```python
from build123d import *

# Parameters (mm, degrees)
SKETCH_W        = 100.5
SKETCH_H        = 50
SKETCH_R        = 19
SKETCH_R_2      = 1.7
SKETCH_W_2      = 20
SKETCH_H_2      = 40
PAD_DEPTH       = 8
SKETCH001_W     = 86.5
SKETCH001_H     = 44
POCKET_DEPTH    = 3
SKETCH002_W     = 96.5
SKETCH002_H     = 2
POCKET001_DEPTH = 4
POCKET002_DEPTH = 2.5
PAD001_DEPTH    = 53
SKETCH005_R     = 1.5
POCKET003_DEPTH = 30
SKETCH006_R     = 1.7
POCKET004_DEPTH = 50.001
POCKET006_DEPTH = 2
FILLET_R        = 3
FILLET001_R     = 3
FILLET002_R     = 3
FILLET003_R     = 3
CHAMFER_SIZE    = 1.6
CHAMFER001_SIZE = 1.6
CHAMFER002_SIZE = 1.6
CHAMFER003_SIZE = 1.6


with BuildPart() as part:
    # Sketch → Pad (new body)
    with BuildSketch(Plane.XY):
        Rectangle(SKETCH_W, SKETCH_H)
        with Locations((23.25, 0)):
            Circle(SKETCH_R, mode=Mode.SUBTRACT)
        with Locations((7.25, 16)):
            Circle(SKETCH_R_2, mode=Mode.SUBTRACT)
        with Locations((39.25, 16)):
            Circle(SKETCH_R_2, mode=Mode.SUBTRACT)
        with Locations((39.25, -16)):
            Circle(SKETCH_R_2, mode=Mode.SUBTRACT)
        with Locations((7.25, -16)):
            Circle(SKETCH_R_2, mode=Mode.SUBTRACT)
        with Locations((-8, 16)):
            Circle(SKETCH_R_2, mode=Mode.SUBTRACT)
        with Locations((-8, -16)):
            Circle(SKETCH_R_2, mode=Mode.SUBTRACT)
        with Locations((-24.25, 0)):
            Rectangle(SKETCH_W_2, SKETCH_H_2, mode=Mode.SUBTRACT)
    extrude(amount=PAD_DEPTH)

    # Sketch001 → Pocket (cut)
    with BuildSketch(Plane.XY.offset(8)):
        Rectangle(SKETCH001_W, SKETCH001_H)
    extrude(amount=-POCKET_DEPTH, mode=Mode.SUBTRACT)

    # Sketch002 → Pocket001 (cut)
    with BuildSketch(Plane.XY.offset(8)):
        with Locations((0, 10.5)):
            Rectangle(SKETCH002_W, SKETCH002_H)
        with Locations((0, -4.5)):
            Rectangle(SKETCH002_W, SKETCH002_H)
    extrude(amount=-POCKET001_DEPTH, mode=Mode.SUBTRACT)

    # Sketch003 → Pocket002 (cut)
    with BuildSketch(Plane.XY.offset(5)):
        Polygon((6.428139, 19.067226), (4.182774, 16.821861), (5.004634, 13.754634), (8.071861, 12.932774), (10.317226, 15.178139), (9.495366, 18.245366), align=None)
        Polygon((40.071861, 19.067226), (37.004634, 18.245366), (36.182774, 15.178139), (38.428139, 12.932774), (41.495366, 13.754634), (42.317226, 16.821861), align=None)
        Polygon((5.004634, -13.754634), (4.182774, -16.821861), (6.428139, -19.067226), (9.495366, -18.245366), (10.317226, -15.178139), (8.071861, -12.932774), align=None)
        Polygon((36.182774, -15.178139), (37.004634, -18.245366), (40.071861, -19.067226), (42.317226, -16.821861), (41.495366, -13.754634), (38.428139, -12.932774), align=None)
        Polygon((-9.587713, 18.75), (-11.175426, 16), (-9.587713, 13.25), (-6.412287, 13.25), (-4.824574, 16), (-6.412287, 18.75), align=None)
        Polygon((-9.587713, -13.25), (-11.175426, -16), (-9.587713, -18.75), (-6.412287, -18.75), (-4.824574, -16), (-6.412287, -13.25), align=None)
    extrude(amount=-POCKET002_DEPTH, mode=Mode.SUBTRACT)

    # Sketch004 → Pad001 (new body)
    with BuildSketch(Plane.XY.offset(8)):
        Polygon((-50.25, 25), (50.25, 25), (50.25, 17), (43.25, 17), (43.25, 22), (-43.25, 22), (-43.25, 17), (-50.25, 17), align=None)
        Polygon((50.25, -17), (50.25, -25), (-50.25, -25), (-50.25, -17), (-43.25, -17), (-43.25, -22), (43.25, -22), (43.25, -17), align=None)
    extrude(amount=PAD001_DEPTH)

    # Sketch005 → Pocket003 (cut)
    with BuildSketch(Plane.XY.offset(61)):
        with Locations((-47, 21)):
            Circle(SKETCH005_R)
        with Locations((47, 21)):
            Circle(SKETCH005_R)
        with Locations((47, -21)):
            Circle(SKETCH005_R)
        with Locations((-47, -21)):
            Circle(SKETCH005_R)
    extrude(amount=-POCKET003_DEPTH, mode=Mode.SUBTRACT)

    # Sketch006 → Pocket004 (cut, through all)
    with BuildSketch(Plane(origin=(0, 25, 0), x_dir=(-1, 0, 0), z_dir=(0, 1, 0))):
        with Locations((-18, 20)):
            Circle(SKETCH006_R)
        with Locations((18, 20)):
            Circle(SKETCH006_R)
        with Locations((-18, 40)):
            Circle(SKETCH006_R)
        with Locations((18, 40)):
            Circle(SKETCH006_R)
    extrude(amount=-POCKET004_DEPTH, mode=Mode.SUBTRACT)

    # Sketch008 → Pocket006 (cut)
    with BuildSketch(Plane(origin=(0, -22, 0), x_dir=(-1, 0, 0), z_dir=(0, 1, 0))):
        Polygon((-14.824574, 20), (-16.412287, 22.75), (-19.587713, 22.75), (-21.175426, 20), (-19.587713, 17.25), (-16.412287, 17.25), align=None)
        Polygon((21.175426, 20), (19.587713, 22.75), (16.412287, 22.75), (14.824574, 20), (16.412287, 17.25), (19.587713, 17.25), align=None)
        Polygon((-16.412287, 37.25), (-14.824574, 40), (-16.412287, 42.75), (-19.587713, 42.75), (-21.175426, 40), (-19.587713, 37.25), align=None)
        Polygon((19.587713, 37.25), (21.175426, 40), (19.587713, 42.75), (16.412287, 42.75), (14.824574, 40), (16.412287, 37.25), align=None)
    extrude(amount=-POCKET006_DEPTH, mode=Mode.SUBTRACT)

    # Fillet
    fillet_edges = [part.edges().sort_by_distance(p)[0] for p in [
        (-50.25, 25, 34.5),
    ]]
    fillet(fillet_edges, radius=FILLET_R)

    # Fillet001
    fillet001_edges = [part.edges().sort_by_distance(p)[0] for p in [
        (-50.25, -25, 34.5),
    ]]
    fillet(fillet001_edges, radius=FILLET001_R)

    # Fillet002
    fillet002_edges = [part.edges().sort_by_distance(p)[0] for p in [
        (50.25, 25, 34.5),
    ]]
    fillet(fillet002_edges, radius=FILLET002_R)

    # Fillet003
    fillet003_edges = [part.edges().sort_by_distance(p)[0] for p in [
        (50.25, -25, 34.5),
    ]]
    fillet(fillet003_edges, radius=FILLET003_R)

    # Chamfer
    chamfer_edges = [part.edges().sort_by_distance(p)[0] for p in [
        (19.7, 22, 40),
    ]]
    chamfer(chamfer_edges, length=CHAMFER_SIZE)

    # Chamfer001
    chamfer001_edges = [part.edges().sort_by_distance(p)[0] for p in [
        (-16.3, 22, 40),
    ]]
    chamfer(chamfer001_edges, length=CHAMFER001_SIZE)

    # Chamfer002
    chamfer002_edges = [part.edges().sort_by_distance(p)[0] for p in [
        (-16.3, 22, 20),
    ]]
    chamfer(chamfer002_edges, length=CHAMFER002_SIZE)

    # Chamfer003
    chamfer003_edges = [part.edges().sort_by_distance(p)[0] for p in [
        (19.7, 22, 20),
    ]]
    chamfer(chamfer003_edges, length=CHAMFER003_SIZE)


solid = part.part
```
Source: CAD feature listing. Evaluate the final solid. Frame: model axes, mm. A direction names the side the tool comes from. Round coordinates to 2 decimals unless told otherwise and drop trailing zeros. Write each loop counter-clockwise with the first axis right and the second up, starting at its lowest first coordinate (ties: lowest second). Pieces come first, ordered by that corner, then holes. Notation, with made-up numbers: M -8,-0.75 L 23,-0.75 A32 cw 23,34.25 Z; hole C 50,55 d11. An arc over 180 degrees is marked long. Use CSV: the item, a comma, the result in double quotes. Start each with the question number.
Q1. Line query: line 1 (X direction, y = 5.5, z = 3.5); line 2 (Y direction, x = -8, z = 1.85); line 3 (Y direction, x = 7.25, z = 1.4). Output: solid intervals per line, ascending. Write a range as from..to.
Q2. Cut plane B-B on x = -32. Output: boundary loops of the cut face in (y, z).
Q3. Cut plane C-C on z = 13.5. Output: boundary loops of the cut face in (x, y).
Q4. Access query for faces 1 (the face through (18, -23, 17.25)), 2 (the face through (-43.25, 19, 33)), 3 (the face through (47, -17, 34)), 4 (the face through (17.2, -24.5, 38.5)). Directions: +Z, -Z, +X, -X, +Y, -Y. A direction counts if a zero-diameter tool reaches every point of the face in a straight line with its end or side. Return the directions, or none.
Q5. Cut plane D-D on x = -8. Count the separate pieces of the cut face and the enclosed holes in it, plus the area to 4 significant figures.
Q6. First-contact query: P1, Ø3.5, axis at x = -46, y = -5, coming from the +Z side; P2, Ø4.5, axis at x = -7.5, y = -16, coming from the +Z side. Flat tips, straight axial feed; report the tip coordinate or a pass-through.
Q7. Pull-direction query (Y, two-part tool) for faces 5 (the face through (-18.8, 24.3, 38.5)), 6 (the face through (-41, -4, 4)); classes: +Y half, -Y half, draft (parallel to the pull), parting line (faces both ways), or undercut.
Q8. Cut plane A-A on z = 33. Output: boundary loops of the cut face in (x, y), plus the area to 3 significant figures.
Results found:
1,line 1,"-50.25..-34.25, -14.25..5.06, 41.44..50.25"
1,line 2,"-25..-17.7, -14.3..14.3, 17.7..25"
1,line 3,"-25..-17.7, -14.3..-10.25, 10.25..14.3, 17.7..25"
2,outline,"M -25,0 L -20,0 L -20,5 L -22,5 L -22,61 L -25,61 Z; M 20,0 L 25,0 L 25,61 L 22,61 L 22,5 L 20,5 Z"
3,outline,"M -50.25,-22 A3 ccw -47.25,-25 L 47.25,-25 A3 ccw 50.25,-22 L 50.25,-17 L 43.25,-17 L 43.25,-22 L -43.25,-22 L -43.25,-17 L -50.25,-17 Z; M -50.25,17 L -43.25,17 L -43.25,22 L 43.25,22 L 43.25,17 L 50.25,17 L 50.25,22 A3 ccw 47.25,25 L -47.25,25 A3 ccw -50.25,22 Z"
4,face 1,"none"
4,face 2,"+Z"
4,face 3,"+Z, +X, -X"
4,face 4,"+Y, -Y"
5,separate pieces,"3"
5,enclosed holes,"0"
5,area,"537.5 mm^2"
6,P1,"z = 8"
6,P2,"z = 2.5"
7,face 5,"draft"
7,face 6,"undercut"
8,outline,"M -50.25,-22 A3 ccw -47.25,-25 L 47.25,-25 A3 ccw 50.25,-22 L 50.25,-17 L 43.25,-17 L 43.25,-22 L -43.25,-22 L -43.25,-17 L -50.25,-17 Z; M -50.25,17 L -43.25,17 L -43.25,22 L 43.25,22 L 43.25,17 L 50.25,17 L 50.25,22 A3 ccw 47.25,25 L -47.25,25 A3 ccw -50.25,22 Z; hole C -47,-21 d3; hole C -47,21 d3; hole C 47,-21 d3; hole C 47,21 d3"
8,area,"707 mm^2"
